from build123d import *

# Parameters (mm, degrees)
BOSS_EXTRUDE1_DEPTH     = 65
CUT_EXTRUDE1_DEPTH      = 183.971935996
CUT_EXTRUDE1_DEPTH_BACK = 183.971935996
CUT_EXTRUDE2_DEPTH      = 183.971935996
CUT_EXTRUDE2_DEPTH_BACK = 183.971935996
SHELL2_T                = -1.5
BOSS_EXTRUDE4_DEPTH     = 5
FILLET12_R              = 10


with BuildPart() as part:
    # Sketch1 → Boss-Extrude1 (new body)
    with BuildSketch(Plane(origin=(0, 0, 0), x_dir=(0, 0, -1), z_dir=(1, 0, 0))):
        with BuildLine():
            Line((-101.278568247, 0), (168.721431753, 0))
            Line((168.721431753, 0), (168.721431753, 14))
            Line((168.721431753, 14), (-66.798599974, 28.050095))
            ThreePointArc((-66.798599974, 28.050095), (-88.293376402, 19.255158243), (-101.278568247, 0))
        make_face()
    extrude(amount=BOSS_EXTRUDE1_DEPTH)

    # Sketch3 → Cut-Extrude1 (cut, two sides: drawn at the far end of the back side and taken through both)
    with BuildSketch(Plane.XZ.offset(-CUT_EXTRUDE1_DEPTH_BACK)):
        Polygon((-75.150987408, 530.638325694), (0, -21.721431753), (20, -168.721431753), (95.150987408, -721.081189199), (-1009.568527485, -871.383164014), (-1179.8705023, 380.336350878), align=None)
    extrude(amount=CUT_EXTRUDE1_DEPTH + CUT_EXTRUDE1_DEPTH_BACK, mode=Mode.SUBTRACT)

    # Sketch5 → Cut-Extrude2 (cut, two sides: drawn at the far end of the back side and taken through both)
    with BuildSketch(Plane.XZ.offset(-CUT_EXTRUDE2_DEPTH_BACK)):
        Polygon((140.150987408, 530.638325694), (65, -21.721431753), (45, -168.721431753), (-30.150987408, -721.081189199), (1074.568527485, -871.383164014), (1244.8705023, 380.336350878), align=None)
    extrude(amount=CUT_EXTRUDE2_DEPTH + CUT_EXTRUDE2_DEPTH_BACK, mode=Mode.SUBTRACT)

    # Shell2
    shell2_openings = [part.faces().sort_by_distance(p)[0] for p in [
        (32.5, 22.000053007, -34.617517295),
        (32.5, 19.255158243, 88.293376402),
    ]]
    offset(amount=SHELL2_T, openings=shell2_openings, kind=Kind.INTERSECTION)

    # Sketch18 → Boss-Extrude4 (add)
    with BuildSketch(Plane.XZ):
        Polygon((65, 101.278568247), (0, 101.278568247), (0, -21.721431753), (20, -168.721431753), (45, -168.721431753), (65, -21.721431753), align=None)
    extrude(amount=BOSS_EXTRUDE4_DEPTH)

    # Fillet12
    fillet12_edges = [part.edges().sort_by_distance(p)[0] for p in [
        (65, -5, 39.778568247),
        (0, -5, 39.778568247),
        (10, -5, -95.221431753),
        (55, -5, -95.221431753),
    ]]
    fillet(fillet12_edges, radius=FILLET12_R)


solid = part.part
The model under review builds one solid part; all positions refer to its coordinate system, in mm. A direction names the side the tool comes from. Coordinates: 2 decimals unless noted, no trailing zeros. Loops run counter-clockwise (first coordinate to the right, second up) from the corner with the lowest first, then second, coordinate; pieces in that order, holes last. Notation, with made-up numbers: (74, 31.5) -> (103, 31.5) arc R13 ccw to (103, 37.5) -> close; hole circle Ø3 at (-29.75, 44). An arc over 180 degrees is marked (long way). Use a Markdown table: item, result. Add a question column.
1. Clearance check with flat-ended pins moving along their axes: pin 1 Ø14 at (x, y) = (35.5, 9.5) entering from +Z; pin 2 Ø12 at (x, z) = (49, -82.5) entering from -Y; pin 3 Ø4 at (y, z) = (0, 5.5) entering from +X; pin 4 Ø12 at (y, z) = (8, -54.5) entering from +X. State where each tip first meets the part, or that it passes through.
2. To check wall thickness, follow line 1 (X direction, y = 5, z = 14); line 2 (Z direction, x = 29.5, y = 12.5); line 3 (Y direction, x = 39, z = 48). State the ranges of each line that lie inside material, in increasing order.
3. Add section C-C on y = 9. Write out the cut boundary in (x, z), plus the area to 3 significant figures.
4. Add section D-D on z = 19. Write out the cut boundary in (x, y), plus the area to 3 significant figures.
5. Add section B-B on z = 84. Write out the cut boundary in (x, y).
6. Machinability: for faces 4 (the face through (32, 8, -167.221)), 5 (the face through (32, 5, -168.721)), which of the approach directions +Z, -Z, +X, -X, +Y, -Y give a long, thin tool a straight path to every point of the face, cutting with its end or side? Answer none if there is none.
7. Draft analysis for pull direction X (two halves, no side actions). For faces 1 (the face through (1.5, 12, 40)), 2 (the face through (2.85, -1.99, 38.92)), 3 (the face through (32, -5, -2)), state which applies: pulls with the +X half, pulls with the -X half, needs draft (parallel to the pull), parting line crosses it, or undercut.
8. Add section A-A on y = 25.5. Write out the cut boundary in (x, z).
Returned:
| question | item | result |
|---|---|---|
| 1 | pin 1 | stops at z = -167.22 |
| 1 | pin 2 | stops at y = -5 |
| 1 | pin 3 | stops at x = 64.54 |
| 1 | pin 4 | stops at x = 61.36 |
| 2 | line 1 | x = 0 to 1.5, 63.5 to 65 |
| 2 | line 2 | z = -168.72 to -167.22 |
| 2 | line 3 | y = -5 to 1.5 |
| 3 | outline | (0, -21.72) -> (20, -168.72) -> (45, -168.72) -> (65, -21.72) -> (65, 97.23) -> (63.5, 97.23) -> (63.5, -21.62) -> (43.69, -167.22) -> (21.31, -167.22) -> (1.5, -21.62) -> (1.5, 97.23) -> (0, 97.23) -> close |
| 3 | area | 835 mm² |
| 4 | outline | (0, 5) arc R10 ccw to (10, -5) -> (55, -5) arc R10 ccw to (65, 5) -> (65, 25.2) -> (63.5, 25.2) -> (63.5, 1.5) -> (1.5, 1.5) -> (1.5, 25.2) -> (0, 25.2) -> close |
| 4 | area | 451 mm² |
| 5 | outline | (0, 5) arc R10 ccw to (10, -5) -> (55, -5) arc R10 ccw to (65, 5) -> (65, 22.3) -> (63.5, 22.3) -> (63.5, 1.5) -> (1.5, 1.5) -> (1.5, 22.3) -> (0, 22.3) -> close |
| 6 | face 4 | +Z, +Y |
| 6 | face 5 | -Z, +X, -X, +Y, -Y |
| 7 | face 1 | undercut |
| 7 | face 2 | pulls with the -X half |
| 7 | face 3 | needs draft |
| 8 | outline | (0, 24.05) -> (1.5, 24.05) -> (1.5, 77.56) -> (0, 77.56) -> close; (63.5, 24.05) -> (65, 24.05) -> (65, 77.56) -> (63.5, 77.56) -> close |
